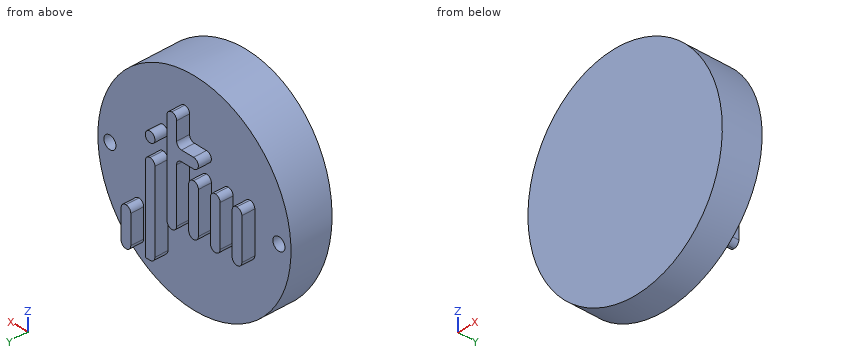
from build123d import *

# Parameters (mm, degrees)
BOSS_EXTRUDE2_DEPTH       = 2.5
SKETCH1_R                 = 1
BOSS_EXTRUDE2_2_DEPTH     = 2.5
SKETCH1_W                 = 2
SKETCH1_H                 = 17.5
BOSS_EXTRUDE2_3_DEPTH     = 2.5
SKETCH1_H_2               = 10
BOSS_EXTRUDE2_4_DEPTH     = 2.5
BOSS_EXTRUDE2_5_DEPTH     = 2.5
BOSS_EXTRUDE2_6_DEPTH     = 2.5
SKETCH1_H_3               = 7.5
BOSS_EXTRUDE2_7_DEPTH     = 2.5
SKETCH1_6_R               = 20
BOSS_EXTRUDE3_DEPTH       = 20
CUT_EXTRUDE1_START        = -27.5000001
CUT_EXTRUDE1_DEPTH        = 40.0000001
FILLET1_R                 = 1
M3X0_5_TAPPED_HOLE1_D     = 2.5
M3X0_5_TAPPED_HOLE1_DEPTH = 2.7
M3X0_5_TAPPED_HOLE1_TIP   = 0.751075774


# Read off the part's stored shape, not the designer's step: Cut-Extrude1
with BuildPart() as part:
    # Sketch1 → Boss-Extrude2 (new body)
    with BuildSketch(Plane(origin=(0, 0, 0), x_dir=(1, 0, 0), z_dir=(0, 1, 0))):
        with BuildLine():
            Line((-2, -20), (0, -20))
            Line((0, -20), (0, 0))
            Line((0, 0), (-2, 0))
            Line((-2, 0), (-2, -12.5))
            Line((-2, -12.5), (-5.5, -12.5))
            ThreePointArc((-5.5, -12.5), (-6.5, -13.5), (-5.5, -14.5))
            Line((-5.5, -14.5), (-2, -14.5))
            Line((-2, -14.5), (-2, -20))
        make_face()
    extrude(amount=BOSS_EXTRUDE2_DEPTH)



with BuildPart() as body_2:
    # Sketch1 → Boss-Extrude2 2 (new body)
    with BuildSketch(Plane(origin=(0, 0, 0), x_dir=(1, 0, 0), z_dir=(0, 1, 0))):
        with Locations(Location((3.5, -13.5, 0), (0, 0, 270))):
            Circle(SKETCH1_R)
    extrude(amount=BOSS_EXTRUDE2_2_DEPTH)


with BuildPart() as body_3:
    # Sketch1 → Boss-Extrude2 3 (new body)
    with BuildSketch(Plane(origin=(0, 0, 0), x_dir=(1, 0, 0), z_dir=(0, 1, 0))):
        with Locations((3.5, -1.25)):
            Rectangle(SKETCH1_W, SKETCH1_H)
    extrude(amount=BOSS_EXTRUDE2_3_DEPTH)


with BuildPart() as body_4:
    # Sketch1 → Boss-Extrude2 4 (new body)
    with BuildSketch(Plane(origin=(0, 0, 0), x_dir=(1, 0, 0), z_dir=(0, 1, 0))):
        with Locations((-5.5, -5.5)):
            Rectangle(SKETCH1_W, SKETCH1_H_2)
    extrude(amount=BOSS_EXTRUDE2_4_DEPTH)


with BuildPart() as body_5:
    # Sketch1 → Boss-Extrude2 5 (new body)
    with BuildSketch(Plane(origin=(0, 0, 0), x_dir=(1, 0, 0), z_dir=(0, 1, 0))):
        with Locations((-10, -5.5)):
            Rectangle(SKETCH1_W, SKETCH1_H_2)
    extrude(amount=BOSS_EXTRUDE2_5_DEPTH)


with BuildPart() as body_6:
    # Sketch1 → Boss-Extrude2 6 (new body)
    with BuildSketch(Plane(origin=(0, 0, 0), x_dir=(1, 0, 0), z_dir=(0, 1, 0))):
        with Locations((-14.5, -5.5)):
            Rectangle(SKETCH1_W, SKETCH1_H_2)
    extrude(amount=BOSS_EXTRUDE2_6_DEPTH)


with BuildPart() as body_7:
    # Sketch1 → Boss-Extrude2 7 (new body)
    with BuildSketch(Plane(origin=(0, 0, 0), x_dir=(1, 0, 0), z_dir=(0, 1, 0))):
        with Locations((8.5, 4.25)):
            Rectangle(SKETCH1_W, SKETCH1_H_3)
    extrude(amount=BOSS_EXTRUDE2_7_DEPTH)


with BuildPart() as part_1:
    add(part.part)

    add(body_2.part)  # Boss-Extrude3 merges body 2

    add(body_3.part)  # Boss-Extrude3 merges body 3

    add(body_4.part)  # Boss-Extrude3 merges body 4

    add(body_5.part)  # Boss-Extrude3 merges body 5

    add(body_6.part)  # Boss-Extrude3 merges body 6

    add(body_7.part)  # Boss-Extrude3 merges body 7
    # Sketch1<6> → Boss-Extrude3 (add)
    with BuildSketch(Plane(origin=(0, 0, 0), x_dir=(1, 0, 0), z_dir=(0, 1, 0))):
        with Locations(Location((-3, -6, 0), (0, 0, 270))):
            Circle(SKETCH1_6_R)
    extrude(amount=-BOSS_EXTRUDE3_DEPTH)

    # Cut-Extrude1 outline → Cut-Extrude1 (cut)
    with BuildSketch(Plane(origin=(4.5, 0, 0), x_dir=(0, 0, -1), z_dir=(1, 0, 0)).offset(CUT_EXTRUDE1_START)):
        Polygon((14, -20), (14, -5.697915295), (-26, -9.902084705), (-26, -20), align=None)
    extrude(amount=CUT_EXTRUDE1_DEPTH, mode=Mode.SUBTRACT)

    # Fillet1
    fillet1_edges = [part_1.edges().sort_by_distance(p)[0] for p in [
        (-13.5, 1.25, 10.5),
        (-13.5, 1.25, 0.5),
        (-9, 1.25, 0.5),
        (-9, 1.25, 10.5),
        (-4.5, 1.25, 0.5),
        (-4.5, 1.25, 10.5),
        (0, 1.25, 20),
        (0, 1.25, 0),
        (9.5, 1.25, -8),
        (9.5, 1.25, -0.5),
        (4.5, 1.25, 10),
        (-15.5, 1.25, 0.5),
        (-15.5, 1.25, 10.5),
        (-11, 1.25, 0.5),
        (-11, 1.25, 10.5),
        (-6.5, 1.25, 0.5),
        (-6.5, 1.25, 10.5),
        (7.5, 1.25, -0.5),
        (7.5, 1.25, -8),
        (2.5, 1.25, -7.5),
        (2.5, 1.25, 10),
        (-2, 1.25, 0),
        (-2, 1.25, 14.5),
        (-2, 1.25, 20),
        (-2, 1.25, 12.5),
    ]]
    fillet(fillet1_edges, radius=FILLET1_R - 0.0001)  # a hair under: the kernel refuses the full size

    # M3x0.5 Tapped Hole1
    with Locations(Plane(origin=(14.5, 0, 6), x_dir=(0, 0, 1), z_dir=(0, 1, 0))):
        with Locations((0, 0), (0, -35)):
            Hole(M3X0_5_TAPPED_HOLE1_D / 2, depth=M3X0_5_TAPPED_HOLE1_DEPTH)
            with Locations((0, 0, -(M3X0_5_TAPPED_HOLE1_DEPTH + M3X0_5_TAPPED_HOLE1_TIP / 2))):  # 118° drill point
                Cone(0, M3X0_5_TAPPED_HOLE1_D / 2, M3X0_5_TAPPED_HOLE1_TIP, mode=Mode.SUBTRACT)


solid = part_1.part
Could you check a few things on this model? Use its own coordinates, in mm. Coordinates: 2 decimals unless noted, no trailing zeros. Order: outer loops, then holes, each group sorted by start corner. A loop starts at its lowest first (then second) coordinate and runs counter-clockwise, first axis right, second up.
Q1. Suppose I cut it at D-D on x = 12.5. Please give me the cut outline in (y, z).
Q2. Please list where these lines run through material, in increasing order: L1, parallel to X at y = -2, z = 6; L2, parallel to X at y = 2, z = -6.5; L3, parallel to Y at x = 3, z = 8.
Q3. Suppose I cut it at C-C on y = -5. Please give me the cut outline in (x, z), and give its area (3 significant figures).
Q4. Will these pins go through, and if not, where does the flat tip stop? pin 1 (3 mm diameter, centred on x = -20.5, z = 6, fed in from +Y); pin 2 (1.2 mm diameter, centred on y = 1, z = -3.5, fed in from -X); pin 3 (1.2 mm diameter, centred on y = 1.5, z = 9.5, fed in from +X); pin 4 (3 mm diameter, centred on x = -4, y = 0.5, fed in from +Z).
Q5. Suppose I cut it at B-B on x = -4. Please give me the cut outline in (y, z).
Q6. Suppose I cut it at A-A on y = 1.25. Give the number of separate pieces and of enclosed holes in the cut face, and give its area (3 significant figures).
Answer:
1. outline: (-9.13, 18.64) - (-6.47, -6.64) - (0, -6.64) - (0, 18.64) - close
2. L1: x = -23 to -21.75, -19.25 to 13.25, 15.75 to 17
2. L2: x = 2.5 to 4.5, 7.5 to 9.5
2. L3: y = -8.01 to 2.5
3. outline: circle Ø40 at (-3, 6)
3. area: 1,260 mm2
4. pin 1: stops at y = 0
4. pin 2: stops at x = 2.5
4. pin 3: stops at x = 4.5
4. pin 4: stops at z = 26
5. outline: (-9.9, 25.97) - (-5.7, -13.97) - (0, -13.97) - (0, 12.5) - (2.5, 12.5) - (2.5, 14.5) - (0, 14.5) - (0, 25.97) - close
6. separate pieces: 7
6. enclosed holes: 0
6. area: 157 mm2
